```python
from build123d import *

# Parameters (mm, degrees)
SKETCH_W            = 110
SKETCH_H            = 28
PAD_DEPTH           = 2.5
SKETCH001_R         = 2.9
PAD001_DEPTH        = 3
SKETCH002_R         = 1
POCKET_DEPTH        = 5.501
POCKET001_DEPTH     = 2.501
LINEARPATTERN_COUNT = 2
LINEARPATTERN_PITCH = 16
SKETCH004_W         = 20
SKETCH004_H         = 10
POCKET002_DEPTH     = 2.501
FILLET_R            = 3.5


with BuildPart() as part:
    # Sketch → Pad (new body)
    with BuildSketch(Plane.XY):
        with Locations((55, 14)):
            Rectangle(SKETCH_W, SKETCH_H)
    extrude(amount=PAD_DEPTH)

    # Sketch001 (on Face6 of Pad) → Pad001 (join)
    with BuildSketch(Plane.XY.offset(2.5)):
        with Locations((15, 24.5)):
            Circle(SKETCH001_R)
        with Locations((73, 24.5)):
            Circle(SKETCH001_R)
    extrude(amount=PAD001_DEPTH)

    # Sketch002 (on Face9 of Pad001) → Pocket (cut, through all)
    with BuildSketch(Plane.XY.offset(5.5)):
        with Locations((15, 24.5)):
            Circle(SKETCH002_R)
        with Locations((73, 24.5)):
            Circle(SKETCH002_R)
    extrude(amount=-POCKET_DEPTH, mode=Mode.SUBTRACT)

    # Sketch003 (on Face5 of Pocket) → Pocket001 (cut, through all)
    with BuildSketch(Plane.XY.offset(2.5)):
        with BuildLine():
            ThreePointArc((29, 4), (25, 0), (29, -4))
            Line((29, -4), (101, -4))
            ThreePointArc((101, -4), (105, 0), (101, 4))
            Line((29, 4), (101, 4))
        make_face()
    pocket001 = extrude(amount=-POCKET001_DEPTH, mode=Mode.SUBTRACT)

    # LinearPattern: Pocket001 ×2
    with Locations(*[(0, i * LINEARPATTERN_PITCH, 0) for i in range(1, LINEARPATTERN_COUNT)]):
        add(pocket001, mode=Mode.SUBTRACT)

    # Sketch004 (on Face4 of LinearPattern) → Pocket002 (cut, through all)
    with BuildSketch(Plane.XY.offset(2.5)):
        with Locations((10, 5)):
            Rectangle(SKETCH004_W, SKETCH004_H)
    extrude(amount=-POCKET002_DEPTH, mode=Mode.SUBTRACT)

    # Fillet
    fillet_edges = [part.edges().sort_by_distance(p)[0] for p in [
        (20, 10, 1.25),
        (0, 10, 1.25),
        (0, 28, 1.25),
        (110, 28, 1.25),
    ]]
    fillet(fillet_edges, radius=FILLET_R)

    # Mirrored: part across XZ


with BuildPart() as part_1:
    add(part.part)
    add(part.part.mirror(Plane.XZ))


solid = part_1.part
```
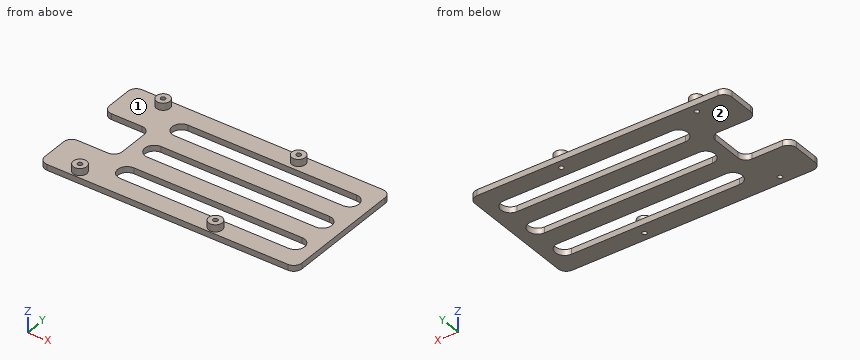
Can you work these out from the model? Positions are in its coordinate system, mm. Face numbers are marked on the shaded views. Give positions to 0.01 mm unless a question says otherwise; leave off trailing zeros. Order: outer loops, then holes, each group sorted by start corner. A loop starts at its lowest first (then second) coordinate and runs counter-clockwise, first axis right, second up. Notation, with made-up numbers: (23, 75) - (68, 75) arc R26 ccw to (68, 92) - close; hole circle Ø2 at (-38.5, 83.25). An arc over 180 degrees is marked (long way). Use a Markdown table: item, result. Add a question column.
Q1. I'm going to push flat-ended pins straight in: pin 1 (6 mm diameter, centred on x = 25.5, y = -19.5, fed in from +Z); pin 2 (3 mm diameter, centred on x = 73, y = 24.5, fed in from -Z); pin 3 (1.2 mm diameter, centred on y = 0, z = 1.5, fed in from -X). Where does each tip first touch, or does it pass through?
Q2. If we section it at C-C on x = 15: Write out the boundary of the cut face in (y, z).
Q3. If we mould it in two halves opening along X, with no side actions, what happens to the marked faces 1 and 2? For each: released by +X, released by -X, zero draft, split by the parting line, or undercut.
Q4. If we section it at D-D on x = 73: Count the separate pieces of the cut face and the enclosed holes in it, plus the area to 3 significant figures.
Q5. If we section it at A-A on z = 3.85: Write out the boundary of the cut face in (x, y).
Q6. If we section it at B-B on y = 0: Write out the boundary of the cut face in (x, z), plus the area to 3 significant figures.
Q7. Please list where these lines run through material, in increasing order: line 1 along Y through (x, z) = (73, 2.55); line 2 along Y through (x, z) = (73, 2.4); line 3 along Y through (x, z) = (15, 2.15).
Answers follow:
| question | item | result |
|---|---|---|
| 1 | pin 1 | stops at z = 2.5 |
| 1 | pin 2 | stops at z = 0 |
| 1 | pin 3 | stops at x = 20 |
| 2 | outline | (-28, 0) - (-25.5, 0) - (-25.5, 5.5) - (-27.4, 5.5) - (-27.4, 2.5) - (-28, 2.5) - close; (-23.5, 0) - (-10, 0) - (-10, 2.5) - (-21.6, 2.5) - (-21.6, 5.5) - (-23.5, 5.5) - close; (10, 0) - (23.5, 0) - (23.5, 5.5) - (21.6, 5.5) - (21.6, 2.5) - (10, 2.5) - close; (25.5, 0) - (28, 0) - (28, 2.5) - (27.4, 2.5) - (27.4, 5.5) - (25.5, 5.5) - close |
| 3 | face 1 | undercut |
| 3 | face 2 | zero draft |
| 4 | separate pieces | 6 |
| 4 | enclosed holes | 0 |
| 4 | area | 92.8 mm^2 |
| 5 | outline | circle Ø5.8 at (15, -24.5); circle Ø5.8 at (15, 24.5); circle Ø5.8 at (73, -24.5); circle Ø5.8 at (73, 24.5); hole circle Ø2 at (15, -24.5); hole circle Ø2 at (15, 24.5); hole circle Ø2 at (73, -24.5); hole circle Ø2 at (73, 24.5) |
| 6 | outline | (20, 0) - (25, 0) - (25, 2.5) - (20, 2.5) - close; (105, 0) - (110, 0) - (110, 2.5) - (105, 2.5) - close |
| 6 | area | 25.0 mm^2 |
| 7 | line 1 | y = -27.4 to -25.5, -23.5 to -21.6, 21.6 to 23.5, 25.5 to 27.4 |
| 7 | line 2 | y = -28 to -25.5, -23.5 to -20, -12 to -4, 4 to 12, 20 to 23.5, 25.5 to 28 |
| 7 | line 3 | y = -28 to -25.5, -23.5 to -10, 10 to 23.5, 25.5 to 28 |
